Autodesk Inventor part; units mm, degrees
ref_plane "YZ Plane" through (0, 0, 0) normal (1, 0, 0) x (0, 1, 0)
ref_plane "XZ Plane" through (0, 0, 0) normal (0, 1, 0) x (-1, 0, 0)
ref_plane "XY Plane" through (0, 0, 0) normal (0, 0, 1) x (1, 0, 0)
sketch "Sketch1" plane through (0, 0, 0) normal (0, 0, 1) x (1, 0, 0)
  circle A0 centre (3.175, -5.4993) radius 1.6764
  circle A1 centre (-3.175, 5.4993) radius 1.6764
  circle A2 centre (0, 0) radius 9.525
  circle A3 centre (-6.35, 0) radius 1.6764
  circle A4 centre (6.35, 0) radius 1.6764
  circle A5 centre (-6.35, 0) radius 1.6764
  circle A6 centre (6.35, 0) radius 1.6764
  point P0 (-9.525, 0)
  point P1 (9.525, 0)
  dimension "d69" = 3.3528
  dimension "d70" = 3.3528
  dimension "d75" = 3.3528
  dimension "d76" = 3.3528
  dimension "d77" = 3.3528
  dimension "d78" = 3.3528
extrude "Extrusion14" add sketch "Sketch1" along normal blind 31.1912
properties part number "Crankshaft"
The listing builds one solid part. Answer for the finished solid, in the listing's coordinates (mm). Coordinates: 2 decimals unless noted, no trailing zeros. Write each loop counter-clockwise with the first axis right and the second up, starting at its lowest first coordinate (ties: lowest second). Pieces come first, ordered by that corner, then holes. Notation, with made-up numbers: (42.5, 30) - (85.5, 30) arc R24 ccw to (85.5, 45) - close; hole circle Ø7 at (-6.75, 66). An arc over 180 degrees is marked (long way). Return JSON: item names as keys, results as strings. Group by question number.
Q1. The part is cut by section A-A on y = 0. Write down the section's boundary in (x, z) (3 decimals), and give its area (3 significant figures).
Q2. For a pull along Y with two mould halves and no side action, classify faces 1 (the cylindrical face through (-7.559, 5.796, 15.377)), 2 (the flat face through (0, 0, 31.191)), 3 (the cylindrical face through (5.02, 1.02, 15.38)) as +Y half, -Y half, draft (parallel to the pull), parting line (faces both ways), or undercut.
Q3. The part is cut by section D-D on z = 4. Write down the section's boundary in (x, y) (3 decimals).
Q4. The part is cut by section B-B on x = -6.35. Write down the section's boundary in (y, z).
Q5. The part is cut by section C-C on y = 6. Write down the section's boundary in (x, z), and give its area (3 significant figures).
Q6. Find the intervals of material crossed by line 1 along X through (y, z) = (1, 4.5); line 2 along Y through (x, z) = (5, 8.5); line 3 along Y through (x, z) = (-6.5, 3), in increasing order. Write a range as [from, to].
Q7. Flat-ended cylindrical pins translate along their axes: pin 1 Ø1.5 at (y, z) = (-4.5, 9.5) entering from +X; pin 2 Ø5 at (y, z) = (3.5, 20) entering from -X; pin 3 Ø2 at (x, z) = (-7.5, 5) entering from +Y. Find the tip coordinate at first contact, or state that the pin passes through.
Evaluation:
{
 "1": {"outline": "(-9.525, 0) - (-8.026, 0) - (-8.026, 31.191) - (-9.525, 31.191) - close; (-4.674, 0) - (4.674, 0) - (4.674, 31.191) - (-4.674, 31.191) - close; (8.026, 0) - (9.525, 0) - (9.525, 31.191) - (8.026, 31.191) - close", "area": "385 mm2"},
 "2": {"face 1": "parting line", "face 2": "draft", "face 3": "undercut"},
 "3": {"outline": "circle Ø19.05 at (0, 0); hole circle Ø3.353 at (-6.35, 0); hole circle Ø3.353 at (-3.175, 5.499); hole circle Ø3.353 at (3.175, -5.499); hole circle Ø3.353 at (6.35, 0)"},
 "4": {"outline": "(-7.1, 0) - (-1.68, 0) - (-1.68, 31.19) - (-7.1, 31.19) - close; (1.68, 0) - (7.1, 0) - (7.1, 31.19) - (1.68, 31.19) - close"},
 "5": {"outline": "(-7.4, 0) - (-4.77, 0) - (-4.77, 31.19) - (-7.4, 31.19) - close; (-1.58, 0) - (7.4, 0) - (7.4, 31.19) - (-1.58, 31.19) - close", "area": "362 mm2"},
 "6": {"line 1": "x = [-9.47, -7.7], [-5, 5], [7.7, 9.47]", "line 2": "y = [-8.11, -0.99], [0.99, 8.11]", "line 3": "y = [-6.96, -1.67], [1.67, 6.96]"},
 "7": {"pin 1": "stops at x = 8.76", "pin 2": "stops at x = -9.47", "pin 3": "stops at y = 6.96"}
}
